The model under review builds one solid part; all positions refer to its coordinate system, in mm. Face numbers are marked on the shaded views. Give positions to 0.01 mm unless a question says otherwise; leave off trailing zeros. Order: outer loops, then holes, each group sorted by start corner. A loop starts at its lowest first (then second) coordinate and runs counter-clockwise, first axis right, second up.
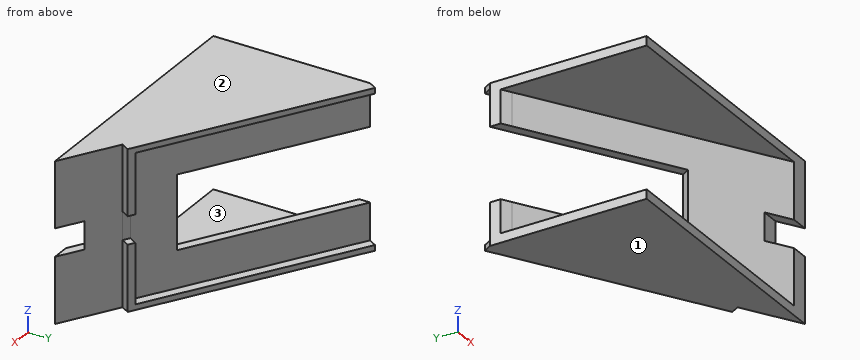
```python
from build123d import *

# Parameters (mm, degrees)
BOSS_EXTRUDE2_DEPTH = 86
BOSS_EXTRUDE3_DEPTH = 5
BOSS_EXTRUDE4_DEPTH = 5
CUT_EXTRUDE2_DEPTH  = 82.06047469
BOSS_EXTRUDE5_DEPTH = 5
CUT_EXTRUDE3_DEPTH  = 6
SKETCH8_W           = 40
SKETCH8_H           = 5.859822581
CUT_EXTRUDE4_DEPTH  = 69.214723926
SKETCH11_W          = 86
SKETCH11_H          = 10
CUT_EXTRUDE6_DEPTH  = 140.082709206
CUT_EXTRUDE8_DEPTH  = 140.082709206
SKETCH14_W          = 15
SKETCH14_H          = 5
CUT_EXTRUDE9_DEPTH  = 10


with BuildPart() as part:
    # Sketch1 → Boss-Extrude2 (new body)
    with BuildSketch(Plane.XY):
        Polygon((0, 89.140177419), (0, 95), (139.082709206, 10), (139.082709206, 0), (0, 0), (0, 5), (5, 5), (134.082709206, 5), (134.082709206, 7.195913121), (5, 86.084441718), align=None)
    extrude(amount=BOSS_EXTRUDE2_DEPTH)

    # Sketch2 → Boss-Extrude3 (add)
    with BuildSketch(Plane.XY.offset(86)):
        Polygon((0, 89.140177419), (134.082709206, 7.195913121), (134.082709206, 5), (0, 5), align=None)
    extrude(amount=-BOSS_EXTRUDE3_DEPTH)

    # Sketch3 → Boss-Extrude4 (add)
    with BuildSketch(Plane(origin=(42.270799685, 69.166321653, 0), x_dir=(0, 0, -1), z_dir=(0.521472393, 0.853268155, 0))):
        Polygon((0, 49.539877301), (0, -78.460122699), (-86, -78.460122699), (-86, 49.539877301), (-83, 49.539877301), (-83, -74.460122699), (-3, -74.460122699), (-3, 49.539877301), align=None)
    extrude(amount=BOSS_EXTRUDE4_DEPTH)

    # Sketch5 → Cut-Extrude2 (cut, through all)
    with BuildSketch(Plane(origin=(42.270799685, 69.166321653, 0), x_dir=(0, 0, -1), z_dir=(0.521472393, 0.853268155, 0))):
        Polygon((-43, 49.539877301), (-23, 49.539877301), (-23, -50.460122699), (-63, -50.460122699), (-63, 49.539877301), align=None)
    extrude(amount=-CUT_EXTRUDE2_DEPTH, mode=Mode.SUBTRACT)

    # Sketch6 → Boss-Extrude5 (add)
    with BuildSketch(Plane(origin=(0, 0, 0), x_dir=(-1, 0, 0), z_dir=(0, 0, -1))):
        Polygon((0, 89.140177419), (-134.082709206, 7.195913121), (-134.082709206, 5), (0, 5), align=None)
    extrude(amount=-BOSS_EXTRUDE5_DEPTH)

    # Sketch7 → Cut-Extrude3 (cut, through all)
    with BuildSketch(Plane(origin=(0, 5, 0), x_dir=(1, 0, 0), z_dir=(0, 1, 0))):
        Polygon((0, -5), (135.193098296, -5), (134.082709206, -81), (0, -81), (0, -63), (62.193208986, -63), (62.193208986, -23), (0, -23), align=None)
    extrude(amount=-CUT_EXTRUDE3_DEPTH, mode=Mode.SUBTRACT)

    # Sketch8 → Cut-Extrude4 (cut, through all)
    with BuildSketch(Plane(origin=(43.056015778, -26.313560917, 0), x_dir=(0, 0, 1), z_dir=(-0.853268155, 0.521472393, 0))):
        with Locations((43, 33.768470979)):
            Rectangle(SKETCH8_W, SKETCH8_H)
    extrude(amount=-CUT_EXTRUDE4_DEPTH, mode=Mode.SUBTRACT)

    # Sketch11 → Cut-Extrude6 (cut, through all)
    with BuildSketch(Plane(origin=(139.082709206, 0, 0), x_dir=(0, 0, -1), z_dir=(1, 0, 0))):
        with Locations((-43, 5)):
            Rectangle(SKETCH11_W, SKETCH11_H)
    extrude(amount=-CUT_EXTRUDE6_DEPTH, mode=Mode.SUBTRACT)

    # Sketch13 → Cut-Extrude8 (cut, through all)
    with BuildSketch(Plane.ZY):
        Polygon((43, 10), (50.5, 10), (50.5, 18), (35.5, 18), (35.5, 10), align=None)
    extrude(amount=-CUT_EXTRUDE8_DEPTH, mode=Mode.SUBTRACT)

    # Sketch14 → Cut-Extrude9 (cut)
    with BuildSketch(Plane(origin=(66.947524108, -40.914787911, 0), x_dir=(0, 0, -1), z_dir=(0.853268155, -0.521472393, 0))):
        with Locations((-43, 83.56047469)):
            Rectangle(SKETCH14_W, SKETCH14_H)
    extrude(amount=-CUT_EXTRUDE9_DEPTH, mode=Mode.SUBTRACT)


solid = part.part
```
1. To check wall thickness, follow line 1 (Z direction, x = 7.5, y = 55); line 2 (X direction, y = 32.5, z = 17); line 3 (X direction, y = 88.5, z = 80). State the ranges of each line that lie inside material, in increasing order.
2. Take a section at D-D (y = 23.5). Write out the cut boundary in (x, z), and give its area (3 significant figures).
3. Insertion check: pin 1 (6 mm diameter, centred on x = 113, z = 66, fed in from -Y); pin 2 (12 mm diameter, centred on x = 70.5, z = 71.5, fed in from -Y); pin 3 (4 mm diameter, centred on x = 19.5, z = 22.5, fed in from +Y); pin 4 (17 mm diameter, centred on x = 56.5, y = 79, fed in from -Z) (3 decimals). Each pin has a flat end and moves straight along its axis. Give the tip position at first contact, or say it passes through.
4. Take a section at C-C (y = 67). Write out the cut boundary in (x, z), and give its area (3 significant figures).
5. Draft analysis for pull direction Z (two halves, no side actions). For the marked faces 1, 2 and 3, state which applies: pulls with the +Z half, pulls with the -Z half, needs draft (parallel to the pull), parting line crosses it, or undercut.
6. Take a section at B-B (z = 58.5). Write out the cut boundary in (x, y), and give its area (3 significant figures).
7. Take a section at A-A (x = 12.5). Write out the cut boundary in (y, z).
Answer:
1. line 1: z = 0 to 5, 81 to 86
1. line 2: x = 92.68 to 102.27, 107.13 to 111.81
1. line 3: x = 1.05 to 10.64
2. outline: (0, 0) - (116.99, 0) - (116.99, 86) - (0, 86) - (0, 81) - (107.4, 81) - (107.4, 5) - (0, 5) - close
2. area: 1,900 mm2
3. pin 1: stops at y = 18.25
3. pin 2: stops at y = 42.39
3. pin 3: stops at y = 84.3
3. pin 4: passes through
4. outline: (0, 0) - (55.4, 0) - (55.4, 3) - (45.82, 3) - (45.82, 23) - (36.23, 23) - (36.23, 5) - (0, 5) - close; (0, 81) - (36.23, 81) - (36.23, 63) - (45.82, 63) - (45.82, 83) - (55.4, 83) - (55.4, 86) - (0, 86) - close
4. area: 861 mm2
5. face 1: pulls with the -Z half
5. face 2: pulls with the +Z half
5. face 3: undercut
6. outline: (82.72, 38.59) - (129.49, 10) - (139.08, 10) - (109.22, 28.25) - (111.83, 32.52) - (108.41, 34.6) - (105.81, 30.34) - (85.33, 42.85) - close
6. area: 315 mm2
7. outline: (10, 0) - (93.22, 0) - (93.22, 3) - (87.36, 3) - (87.36, 23) - (81.5, 23) - (81.5, 5) - (10, 5) - close; (10, 81) - (81.5, 81) - (81.5, 63) - (87.36, 63) - (87.36, 83) - (93.22, 83) - (93.22, 86) - (10, 86) - close
